Input: dimensioned drawing with shaded views. Units: mm. Origin: part minimum x, y, z. Give positions to 0.01 mm unless a question says otherwise; leave off trailing zeros. Order: outer loops, then holes, each group sorted by start corner. A loop starts at its lowest first (then second) coordinate and runs counter-clockwise, first axis right, second up. Notation, with made-up numbers: (-17.5, 30.25) - (23.5, 30.25) arc R28 ccw to (23.5, 55.25) - close; hole circle Ø1 at (72, -37.5). An arc over 180 degrees is marked (long way). Use a Markdown table: item, result.
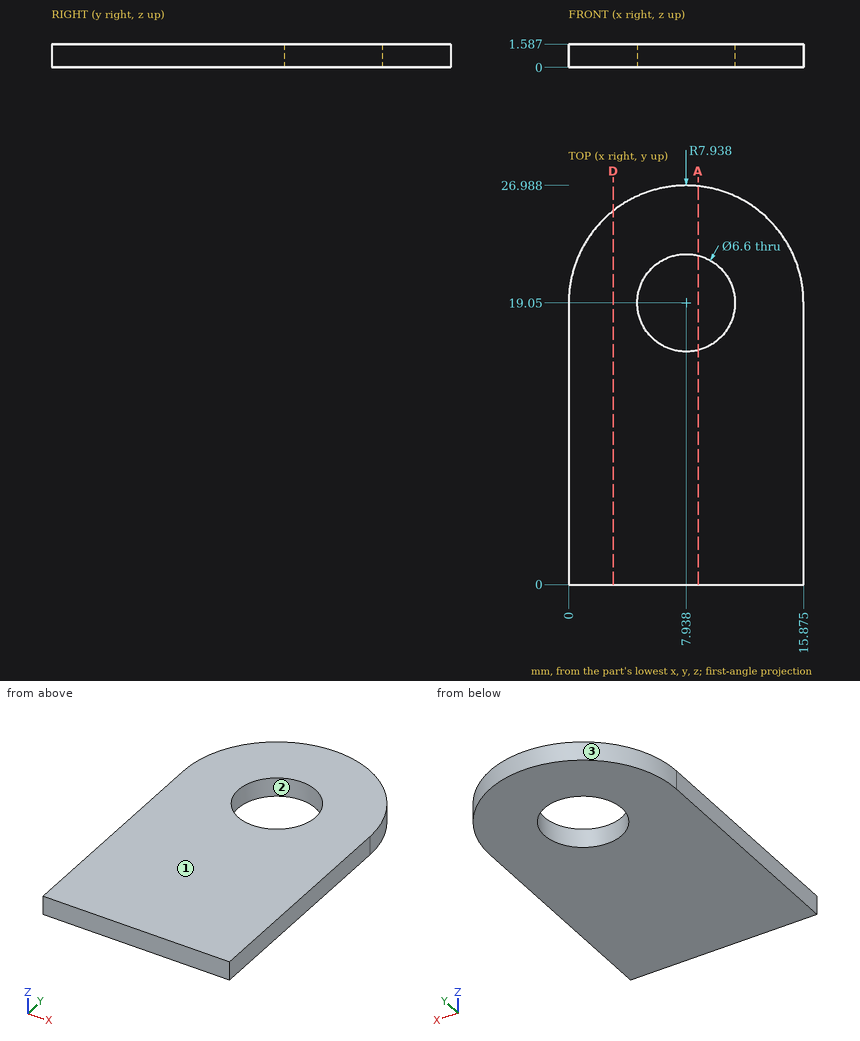
1. Section query A-A (x = 8.75). Return loops of the section in (y, z) (1 decimal).
Response:
| item | result |
|---|---|
| outline | (0, 0) - (15.9, 0) - (15.9, 1.6) - (0, 1.6) - close; (22.2, 0) - (26.9, 0) - (26.9, 1.6) - (22.2, 1.6) - close |
2. Mould query, pull axis X, two halves, no side actions, for the marked faces 1, 2 and 3. Classes: pulls with the +X half, pulls with the -X half, needs draft (parallel to the pull), parting line crosses it, or undercut.
Response:
| item | result |
|---|---|
| face 1 | needs draft |
| face 2 | undercut |
| face 3 | parting line crosses it |
3. Section query D-D (x = 3). Return loops of the section in (y, z) (1 decimal).
Response:
| item | result |
|---|---|
| outline | (0, 0) - (25.3, 0) - (25.3, 1.6) - (0, 1.6) - close |
4. Material intervals for line 1 along Y through (x, z) = (8, 0.7); line 2 along X through (y, z) = (19.5, 0.3); line 3 along Y through (x, z) = (9, 0.8) (1 decimal), sorted ascending.
Response:
| item | result |
|---|---|
| line 1 | y = 0 to 15.75, 22.35 to 26.99 |
| line 2 | x = 0.01 to 4.67, 11.21 to 15.86 |
| line 3 | y = 0 to 15.9, 22.2 to 26.9 |
